```python
from build123d import *

# Parameters (mm, degrees)
F0_R     = 2.5
F1_DEPTH = 2
F2_SIZE  = 0.5
F3_R     = 0.5


with BuildPart() as f1:
    # F0 (on Front) → F1 (new body)
    with BuildSketch(Plane.XZ):
        with BuildLine():
            Line((-2.641257, 12.3198), (-21.641257, 12.3198))
            ThreePointArc((-21.641257, 12.3198), (-28.141257, 5.8198), (-21.641257, -0.6802))
            Line((-21.641257, -0.6802), (-2.641257, -0.6802))
            ThreePointArc((-2.641257, -0.6802), (3.858743, 5.8198), (-2.641257, 12.3198))
        make_face()
        with Locations((-21.641257, 5.8198)):
            Circle(F0_R, mode=Mode.SUBTRACT)
        with Locations((-2.641257, 5.8198)):
            Circle(F0_R, mode=Mode.SUBTRACT)
    extrude(amount=F1_DEPTH)

    # F2
    f2_edges = [f1.edges().sort_by_distance(p)[0] for p in [
        (-24.141257, -2, 5.8198),
        (-5.141257, -2, 5.8198),
        (-5.141257, 0, 5.8198),
        (-24.141257, 0, 5.8198),
    ]]
    chamfer(f2_edges, length=F2_SIZE)

    # F3
    f3_edges = [f1.edges().sort_by_distance(p)[0] for p in [
        (-12.141257, 0, 12.3198),
        (-12.141257, -2, 12.3198),
    ]]
    fillet(f3_edges, radius=F3_R)


solid = f1.part
```
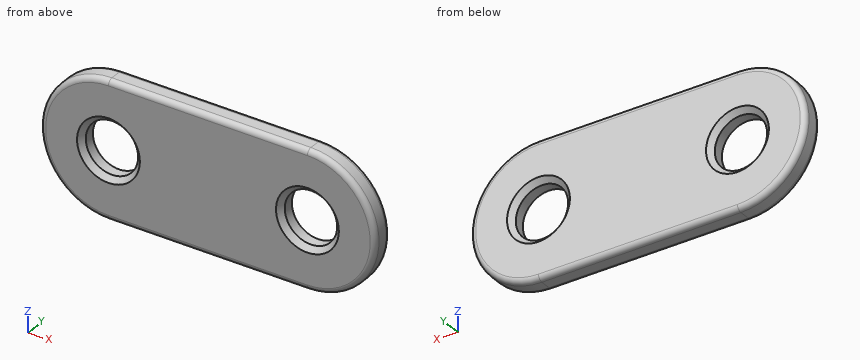
For this review, take the finished solid that the model builds, in its own axes (mm). Round coordinates to 2 decimals unless told otherwise and drop trailing zeros. Write each loop counter-clockwise with the first axis right and the second up, starting at its lowest first coordinate (ties: lowest second). Pieces come first, ordered by that corner, then holes. Notation, with made-up numbers: (45, -13.5) -> (80, -13.5) arc R23 cw to (80, 24.5) -> close; hole circle Ø8 at (86, 18). An arc over 180 degrees is marked (long way). One line per question, with ' | ' between items. Start each with the question number.
(1) Add section B-B, the plane y = -1.1. Write out the cut boundary in (x, z).
(2) For line 1 along X through (y, z) = (-1.4, 7.25); line 2 along X through (y, z) = (-0.9, 7); line 3 along Z through (x, y) = (-4, -1.9), list the stretches that pass through material, from the lowest coordinate up. Write a range as from..to.
(3) Add section A-A, the plane z = 4.5. Give the number of separate pieces and of enclosed holes in the cut face, plus the area to 3 significant figures.
(4) Insertion check: P1, Ø3, axis at x = -2.64, z = 5.82, coming from the -Y side. The pin has a flat end and moves straight along its axis. Give the tip position at first contact, or say it passes through.
Answer list:
1) outline: (-21.64, -0.68) -> (-2.64, -0.68) arc R6.5 ccw to (-2.64, 12.32) -> (-21.64, 12.32) arc R6.5 ccw to start; hole circle Ø5 at (-21.64, 5.82); hole circle Ø5 at (-2.64, 5.82)
2) line 1: -27.98..-23.69, -19.59..-4.69, -0.59..3.7 | line 2: -28.03..-23.85, -19.44..-4.85, -0.44..3.75 | line 3: -0.48..3.26, 8.38..12.12
3) separate pieces: 3 | enclosed holes: 0 | area: 45.1 mm²
4) P1: through
